Could you check a few things on this model? Use its own coordinates, in mm. Face numbers are marked on the shaded views. A direction names the side the tool comes from. Give positions to 0.01 mm unless a question says otherwise; leave off trailing zeros. Write each loop counter-clockwise with the first axis right and the second up, starting at its lowest first coordinate (ties: lowest second). Pieces come first, ordered by that corner, then holes. Notation, with made-up numbers: M 85.5,-31 L 112.5,-31 A23 ccw 112.5,-3 Z; hole C 67.5,87 d8. An arc over 180 degrees is marked long. One line per item, written item: value.
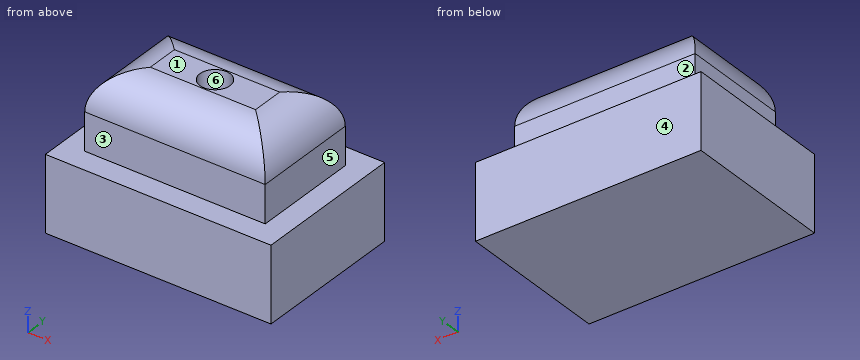
```python
from build123d import *

# Parameters (mm, degrees)
F0_W     = 300
F0_H     = 203.185
F1_DEPTH = 100
F2_W     = 240
F2_H     = 143.185
F3_DEPTH = 100
F4_R     = 50
F5_R     = 20
F6_DEPTH = 170


with BuildPart() as f1:
    # F0 (on Top) → F1 (new body)
    with BuildSketch(Plane.XY):
        with Locations((77.316695, 26.535105)):
            Rectangle(F0_W, F0_H)
    extrude(amount=F1_DEPTH)

    # F2 (on face) → F3 (join)
    with BuildSketch(Plane.XY.offset(100)):
        with Locations((77.316695, 26.535105)):
            Rectangle(F2_W, F2_H)
    extrude(amount=F3_DEPTH)

    # F4
    f4_edges = [f1.edges().sort_by_distance(p)[0] for p in [
        (77.316695, 98.127605, 200),
        (-42.683305, 26.535105, 200),
        (77.316695, -45.057395, 200),
        (197.316695, 26.535105, 200),
    ]]
    fillet(f4_edges, radius=F4_R)

    # F5 (on face) → F6 (cut)
    with BuildSketch(Plane.XY.offset(200)):
        with Locations((77.316695, 26.535105)):
            Circle(F5_R)
    extrude(amount=-F6_DEPTH, mode=Mode.SUBTRACT)


solid = f1.part
```
1) We'd pull the mould along Y, two halves only. Please class the marked faces 3, 4, 5 and 6: pulls with the +Y half, pulls with the -Y half, needs draft (parallel to the pull), parting line crosses it, or undercut.
Outcome:
face 3: pulls with the -Y half
face 4: pulls with the +Y half
face 5: needs draft
face 6: undercut
2) I'm going to push flat-ended pins straight in: pin 1 (10 mm diameter, centred on y = -43.5, z = 117.5, fed in from +X); pin 2 (24 mm diameter, centred on x = 77.32, y = 26.54, fed in from +Z); pin 3 (25 mm diameter, centred on y = 4, z = 134, fed in from -X). Where does each tip first touch, or does it pass through?
Outcome:
pin 1: stops at x = 197.32
pin 2: stops at z = 30
pin 3: stops at x = -42.68
3) If we section it at C-C, the plane y = -25: Write out the boundary of the cut face in (x, z), then the cut area to 3 significant figures.
Outcome:
outline: M -72.68,0 L 227.32,0 L 227.32,100 L 197.32,100 L 197.32,150 A50 ccw 177.26,190.04 L -22.63,190.04 A50 ccw -42.68,150 L -42.68,100 L -72.68,100 Z
area: 51,100 mm^2
4) If we section it at B-B, the plane z = 42: Write out the boundary of the cut face in (x, y).
Outcome:
outline: M -72.68,-75.06 L 227.32,-75.06 L 227.32,128.13 L -72.68,128.13 Z; hole C 77.32,26.54 d40
5) If we section it at A-A, the plane x = 22: Write out the boundary of the cut face in (y, z).
Outcome:
outline: M -75.06,0 L 128.13,0 L 128.13,100 L 98.13,100 L 98.13,150 A50 ccw 48.13,200 L 4.94,200 A50 ccw -45.06,150 L -45.06,100 L -75.06,100 Z
6) On a 3-axis mill with a long thin cutter (end or side, diameter ignored), from which of +Z, -Z, +X, -X, +Y, -Y can I reach the whole of each face in a straight line? I mean the marked faces 1 and 2. Say none if no direction works.
Outcome:
face 1: +Z, +X, -X, +Y, -Y
face 2: +Z, +X, -X, +Y
7) If we section it at D-D, the plane z = 130: Write out the boundary of the cut face in (x, y).
Outcome:
outline: M -42.68,-45.06 L 197.32,-45.06 L 197.32,98.13 L -42.68,98.13 Z; hole C 77.32,26.54 d40
8) Please list where these lines run through material, in increasing order: L1, parallel to Z at x = 163.5, y = 20; L2, parallel to X at y = 83, z = 110.5; L3, parallel to Y at x = 24, z = 105. Write a range as from..to.
Outcome:
L1: z = 0..197.31
L2: x = -42.68..197.32
L3: y = -45.06..98.13
